Autodesk Fusion 360 part; units mm, degrees
sketch "Sketch1" plane through (0, 0, 0) normal (1, 0, 0) x (0, 1, 0) in component "[a]_latch"
  spline S0 degree 3 poles (-10.6277, 6.4557) (-10.4802, 5.6222) (-10.1713, 4.8255) (-9.2656, 3.3954) (-8.6774, 2.7757) (-7.4408, 1.8988) (-6.8381, 1.5983) (-5.5622, 1.1918) (-4.8966, 1.0884) (-4.2271, 1.0884) knots 0 0 0 0 0.253919 0.253919 0.507838 0.507838 0.708696 0.708696 0.909554 0.909554 0.909554 0.909554
  line L0 (-10.6277, 6.4557) -> (-10.4802, 5.6222)
  line L1 (-10.4802, 5.6222) -> (-10.1713, 4.8255)
  line L2 (-10.1713, 4.8255) -> (-9.2656, 3.3954)
  line L3 (-9.2656, 3.3954) -> (-8.6774, 2.7757)
  line L4 (-8.6774, 2.7757) -> (-7.4408, 1.8988)
  line L5 (-7.4408, 1.8988) -> (-6.8381, 1.5983)
  line L6 (-6.8381, 1.5983) -> (-5.5622, 1.1918)
  line L7 (-5.5622, 1.1918) -> (-4.8966, 1.0884)
  line L8 (-4.8966, 1.0884) -> (-4.2271, 1.0884)
  line L9 (-10.6277, 6.4557) -> (-11.487, 11.3114)
  arc A0 (-11.487, 11.3114) -> (-14.4411, 10.7886) centre (-12.964, 11.05) ccw
  line L10 (-14.4411, 10.7886) -> (-14.1338, 9.0523)
  arc A1 (-15.3647, 6.8451) -> (-14.1338, 9.0523) centre (-16.1032, 8.7038) ccw
  arc A2 (-15.3647, 6.8451) -> (-15.5863, -0.7728) centre (-13.8325, 2.9884) ccw
  line L11 (-15.5863, -0.7728) -> (-12.862, -2.0432)
  arc A3 (-12.862, -2.0432) -> (-10.749, -2.5116) centre (-10.749, 2.4884) ccw
  line L12 (-10.749, -2.5116) -> (-2.5005, -2.5116)
  arc A4 (7.6148, -6.4355) -> (-2.5005, -2.5116) centre (-2.5005, -17.5116) ccw
  line L13 (7.6148, -6.4355) -> (12.7434, -11.1193)
  arc A5 (12.7434, -11.1193) -> (14.7665, -8.904) centre (13.7549, -10.0116) ccw
  line L14 (14.7665, -8.904) -> (13.9062, -8.1184)
  arc A6 (13.2549, -6.6416) -> (13.9062, -8.1184) centre (15.2549, -6.6416) ccw
  line L15 (13.2549, -6.6416) -> (13.2549, -0.2086)
  arc A7 (13.9874, 1.3385) -> (13.2549, -0.2086) centre (15.2549, -0.2086) ccw
  arc A8 (13.9874, 1.3385) -> (15.1677, 2.4015) centre (3.2133, 14.4884) ccw
  arc A9 (15.1677, 2.4015) -> (16.3522, 5.0986) centre (12.3549, 5.2455) ccw
  arc A10 (16.3522, 5.0986) -> (15.0788, 6.0971) centre (15.3529, 5.1354) ccw
  arc A11 (11.309, 5.2082) -> (15.0788, 6.0971) centre (3.5545, 46.5367) ccw
  arc A12 (11.309, 5.2082) -> (10.8832, 3.9768) centre (11.4473, 4.4711) ccw
  arc A13 (10.4966, 1.6845) -> (10.8832, 3.9768) centre (9.7549, 2.9884) ccw
  arc A14 (8.3883, 1.0884) -> (10.3175, 1.5843) centre (8.3883, 5.0884) ccw
  arc A15 (10.3175, 1.5843) -> (10.4966, 1.6845) centre (3.2133, 14.4884) ccw
  line L16 (8.3883, 1.0884) -> (-4.2271, 1.0884)
  circle A16 centre (-13.8325, 2.9884) radius 1.75
extrude "Extrude1" add sketch "Sketch1" along normal mid plane 11 in component "[a]_latch"
chamfer "Chamfer1" distance 0.2 angle 45 52 edges at (5.5, -11.0573, 8.8835) (5.5, -13.2254, 12.527) (5.5, -14.2874, 9.9204) (5.5, -14.3565, 7.7296) (5.5, -17.9807, 3.109) (5.5, -14.2242, -1.408) (5.5, -11.8312, -2.3931) (5.5, -6.6247, -2.5116) (5.5, 2.9244, -3.527) (5.5, 10.1791, -8.7774) (5.5, 14.8625, -11.0232) (5.5, 14.3363, -8.5112) (5.5, 13.425, -7.4486) (5.5, 13.2549, -3.4251) (5.5, 13.4473, 0.6473) (5.5, 14.59, 1.8562) (5.5, 16.0173, 3.6371) (5.5, 15.9699, 5.9223) (5.5, 13.2041, 5.6092) (5.5, 10.7385, 4.7162) (5.5, 11.234, 2.7389) (5.5, 10.4072, 1.6341) (5.5, 9.3843, 1.2143) (5.5, 2.0806, 1.0884) (5.5, -8.4061, 2.6098) (5.5, -15.464, 3.6212) (-5.5, -11.0573, 8.8835) (-5.5, -8.4061, 2.6098) (-5.5, 2.0806, 1.0884) (-5.5, 9.3843, 1.2143) (-5.5, 10.4072, 1.6341) (-5.5, 11.234, 2.7389) (-5.5, 10.7385, 4.7162) (-5.5, 13.2041, 5.6092) (-5.5, 15.9699, 5.9223) (-5.5, 16.0173, 3.6371) (-5.5, 14.59, 1.8562) (-5.5, 13.4473, 0.6473) (-5.5, 13.2549, -3.4251) (-5.5, 13.425, -7.4486) (-5.5, 14.3363, -8.5112) (-5.5, 14.8625, -11.0232) (-5.5, 10.1791, -8.7774) (-5.5, 2.9244, -3.527) (-5.5, -6.6247, -2.5116) (-5.5, -11.8312, -2.3931) (-5.5, -14.2242, -1.408) (-5.5, -17.9807, 3.109) (-5.5, -14.3565, 7.7296) (-5.5, -14.2874, 9.9204) (-5.5, -13.2254, 12.527) (-5.5, -15.464, 2.3555) in component "[a]_latch"
sketch "Sketch2" plane through (0, 13.2549, 0) normal (0, 1, 0) x (-1, 0, 0) in component "[a]_latch"
  line L0 (5.3, -6.6416) -> (5.3, -0.2086)
  line L1 (5.3, -0.2086) -> (-5.3, -0.2086)
  line L2 (-5.3, -0.2086) -> (-5.3, -6.6416)
  line L3 (-5.3, -6.6416) -> (5.3, -6.6416)
  line L4 (-1.7321, -1.9251) -> (1.7321, -1.9251)
  line L5 (1.7321, -1.9251) -> (0, -4.9251)
  line L6 (0, -4.9251) -> (-1.7321, -1.9251)
extrude "Extrude2" cut sketch "Sketch2" against normal blind 1 contours L4 L5 L6 in component "[a]_latch"
component "[a]_latch" placed x (1, 0, 0) y (0, 1, 0) z (0, 0, 1) at (0, 0, 0)
Input: part model. Units: mm. Frame: model coordinates. A direction names the side the tool comes from. Give positions to 0.01 mm unless a question says otherwise; leave off trailing zeros. Order: outer loops, then holes, each group sorted by start corner. A loop starts at its lowest first (then second) coordinate and runs counter-clockwise, first axis right, second up. Notation, with made-up numbers: M 63,43.25 L 113,43.25 A14 cw 113,54.25 Z; hole C 56,54.5 d4. An arc over 180 degrees is marked long. Return JSON: item names as keys, results as strings.
1) Line query: L1, parallel to Y at x = 0.25, z = 2.25; L2, parallel to Z at x = -2.75, y = -6.5; L3, parallel to Z at x = -4, y = -2. Output: solid intervals per line, ascending. Write a range as [from, to].
Taken from the geometry:
{"L1": "y = [-17.92, -15.42], [-12.25, -7.94], [11.06, 15.01]", "L2": "z = [-2.51, 1.5]", "L3": "z = [-2.52, 1.09]"}
2) Contact query for flat-ended pins moving along their axis: pin 1 (1.5 mm diameter, centred on x = 3.5, y = -7, fed in from -Z); pin 2 (3 mm diameter, centred on x = 1.5, y = 0.5, fed in from +Z); pin 3 (3 mm diameter, centred on x = -4, y = 0, fed in from -Z). Output: stop coordinate, or through.
Taken from the geometry:
{"pin 1": "stops at z = -2.51", "pin 2": "stops at z = 1.09", "pin 3": "stops at z = -3.05"}
3) Section query A-A on z = -1.25. Output: boundary loops of the cut face in (x, y), and give its area (3 significant figures).
Taken from the geometry:
{"outline": "M -5.5,-14.09 L -5.3,-14.56 L 5.3,-14.56 L 5.5,-14.09 L 5.5,13.05 L 5.3,13.25 L -5.3,13.25 L -5.5,13.05 Z", "area": "306 mm2"}
4) Mould query, pull axis X, two halves, no side actions, for faces 1 (the face through (0, -7, -2.512)), 2 (the face through (0, 12.255, -3)), 3 (the face through (-5.5, 0.4, 0.6)), 4 (the face through (5.5, 0.4, 0.6)). Classes: released by +X, released by -X, zero draft, split by the parting line, or undercut.
Taken from the geometry:
{"face 1": "zero draft", "face 2": "undercut", "face 3": "released by -X", "face 4": "released by +X"}
5) Access query for faces 5 (the face through (-0.07, -14.29, 9.93)), 6 (the face through (-0.074, 10.735, 4.706)), 7 (the face through (0, 13, -1.925)), 8 (the face through (-1.3, 13.255, -3.5)), 9 (the face through (-0.074, 13.231, 5.615)). Directions: +Z, -Z, +X, -X, +Y, -Y. A direction counts if a zero-diameter tool reaches every point of the face in a straight line with its end or side. Return the directions, or none.
Taken from the geometry:
{"face 5": "+X, -X, -Y", "face 6": "+X, -X", "face 7": "+Y", "face 8": "+X, -X, +Y", "face 9": "+Z, +X, -X"}
6) Section query B-B on z = 3.5. Count the separate pieces of the cut face and the enclosed holes in it, and give its area (3 significant figures).
Taken from the geometry:
{"separate pieces": "3", "enclosed holes": "0", "area": "111 mm2"}
